For this review, take the finished solid that the model builds, in its own axes (mm). A direction names the side the tool comes from. Give positions to 0.01 mm unless a question says otherwise; leave off trailing zeros. Order: outer loops, then holes, each group sorted by start corner. A loop starts at its lowest first (then second) coordinate and runs counter-clockwise, first axis right, second up.
Item 1: Consider section A-A (y = 4.5). Give the boundary of the cut face in (x, z).
Item 2: Machinability: for faces 5 (the flat face through (18.133, 7, -34)), 6 (the flat face through (22.895, 7, 9)), 7 (the flat face through (-6, 7, -29.251)), 8 (the flat face through (13, 7, -38.776)), which of the approach directions +Z, -Z, +X, -X, +Y, -Y give a long, thin tool a straight path to every point of the face, cutting with its end or side? Answer none if there is none.
Item 3: Consider section D-D (x = 4). Give the boundary of the cut face in (y, z) (3 decimals), plus the area to 3 significant figures.
Item 4: The part is to be moulded in two halves that separate along X. For faces 1 (the flat face through (-27.905, 0, -14)), 2 (the flat face through (-15.205, 7, 9)), 3 (the flat face through (32.42, 7, 9)), 4 (the flat face through (28, 7, 13.612)), say which applies: released by +X, released by -X, zero draft, split by the parting line, or undercut.
Item 5: Consider section B-B (z = 9). Give the boundary of the cut face in (x, y) (1 decimal), plus the area to 3 significant figures.
Item 6: For probe 1 along Y at (x, z) = (13, -28.5) (3 decimals); probe 2 along Z at (x, y) = (16.5, 8); probe 3 along Z at (x, y) = (-23.5, 9.5), list the stretches that pass through material, from the lowest coordinate up.
Item 7: For P1, Ø8.5, axis at x = 12.5, y = 7.5, coming from the +Z side; P2, Ø5.5, axis at x = 3.85, z = -32.43, coming from the -Y side; P3, Ø4, axis at x = -21, y = 6, coming from the -Z side; P4, Ø8.5, axis at y = 8, z = 7, coming from the +X side, all flat-tipped, find the tip position at first contact; note any pin that passes through.
Item 8: Consider section C-C (x = -17). Give the boundary of the cut face in (y, z) (1 decimal), plus the area to 3 significant figures.
```python
from build123d import *

# Parameters (mm, degrees)
F0_W     = 17.4625
F0_H     = 63.5
F0_R     = 3.175
F0_R_2   = 9.525
F0_W_2   = 21.1666666667
F0_H_2   = 3.175
F1_DEPTH = 3.175
F2_W     = 9.525
F2_H     = 9.525
F3_DEPTH = 7.9375


with BuildPart() as f1:
    # F0 (on Front) → F1 (new body, symmetric)
    with BuildSketch(Plane.XZ):
        Polygon((-10.4423522066, -45.1256732441), (-27.9048522066, -45.1256732441), (-27.9048522066, -48.3006732441), (-6.7381855399, -48.3006732441), (-6.7381855399, -45.1256732441), align=None)
        Polygon((35.5951477934, -45.1256732441), (18.1326477934, -45.1256732441), (14.4284811268, -45.1256732441), (14.4284811268, -48.3006732441), (35.5951477934, -48.3006732441), align=None)
        with Locations((-19.1736022066, -13.3756732441)):
            Rectangle(F0_W, F0_H)
        Polygon((18.1326477934, 18.3743267559), (-10.4423522066, 18.3743267559), (-10.4423522066, -45.1256732441), (-6.7381855399, -45.1256732441), (14.4284811268, -45.1256732441), (18.1326477934, -45.1256732441), align=None)
        with Locations((3.8451477934, -32.4256732441)):
            Circle(F0_R, mode=Mode.SUBTRACT)
        with Locations((3.8451477934, 2.4993267559)):
            Circle(F0_R_2, mode=Mode.SUBTRACT)
        with Locations((26.8638977934, -13.3756732441)):
            Rectangle(F0_W, F0_H)
        with Locations((3.8451477934, -46.7131732441)):
            Rectangle(F0_W_2, F0_H_2)
    extrude(amount=F1_DEPTH, both=True)

    # F2 (on face) → F3 (join)
    with BuildSketch(Plane(origin=(0, 3.175, 0), x_dir=(-1, 0, 0), z_dir=(0, 1, 0))):
        with Locations((19.9673522066, 8.8493267559)):
            Rectangle(F2_W, F2_H)
        with Locations((-27.6576477934, 8.8493267559)):
            Rectangle(F2_W, F2_H)
        with Locations((-13.3701477934, -34.0131732441)):
            Rectangle(F2_W, F2_H)
        with Locations((5.6798522066, -34.0131732441)):
            Rectangle(F2_W, F2_H)
    extrude(amount=F3_DEPTH)


solid = f1.part
```
Resolved:
1. outline: (-24.73, 4.09) - (-15.2, 4.09) - (-15.2, 13.61) - (-24.73, 13.61) - close; (-10.44, -38.78) - (-0.92, -38.78) - (-0.92, -29.25) - (-10.44, -29.25) - close; (8.61, -38.78) - (18.13, -38.78) - (18.13, -29.25) - (8.61, -29.25) - close; (22.9, 4.09) - (32.42, 4.09) - (32.42, 13.61) - (22.9, 13.61) - close
2. face 5: +Z, -Z, +X, +Y
2. face 6: +Z, -Z, +Y
2. face 7: +Z, +X, -X, +Y
2. face 8: -Z, +X, -X, +Y
3. outline: (-3.175, -48.301) - (3.175, -48.301) - (3.175, -35.597) - (-3.175, -35.597) - close; (-3.175, -29.254) - (3.175, -29.254) - (3.175, -7.024) - (-3.175, -7.024) - close; (-3.175, 12.023) - (3.175, 12.023) - (3.175, 18.374) - (-3.175, 18.374) - close
3. area: 262 mm2
4. face 1: released by -X
4. face 2: undercut
4. face 3: released by +X
4. face 4: zero draft
5. outline: (-27.9, -3.2) - (-3.1, -3.2) - (-3.1, 3.2) - (-15.2, 3.2) - (-15.2, 11.1) - (-24.7, 11.1) - (-24.7, 3.2) - (-27.9, 3.2) - close; (10.8, -3.2) - (35.6, -3.2) - (35.6, 3.2) - (32.4, 3.2) - (32.4, 11.1) - (22.9, 11.1) - (22.9, 3.2) - (10.8, 3.2) - close
5. area: 466 mm2
6. probe 1: y = -3.175 to 3.175
6. probe 2: z = -38.78 to -29.25
6. probe 3: z = 4.09 to 13.61
7. P1: stops at z = -29.25
7. P2: passes through
7. P3: stops at z = 4.09
7. P4: stops at x = 32.42
8. outline: (-3.2, -48.3) - (3.2, -48.3) - (3.2, 4.1) - (11.1, 4.1) - (11.1, 13.6) - (3.2, 13.6) - (3.2, 18.4) - (-3.2, 18.4) - close
8. area: 499 mm2
